Could you check a few things on this model? Use its own coordinates, in mm. Round coordinates to 2 decimals unless told otherwise and drop trailing zeros. Order: outer loops, then holes, each group sorted by start corner. A loop starts at its lowest first (then second) coordinate and runs counter-clockwise, first axis right, second up. Notation, with made-up numbers: M 24,11 L 31,11 A18 cw 31,22 Z; hole C -38,31.25 d11. An arc over 180 degrees is marked long. Write each question's results on one line, items separated by ' | '. Start each with the question number.
1. Suppose I cut it at D-D on x = 28. Write out the boundary of the cut face in (y, z).
2. We'd pull the mould along Z, two halves only. Please class faces 1 (the flat face through (15, -1.626, -13)), 2 (the flat face through (59.822, 0.023, 34.384)), 3 (the cylindrical face through (-11.59, 0.02, -15.12)): released by +Z, released by -Z, zero draft, split by the parting line, or undercut.
3. Please list where these lines run through material, in increasing order: L1, parallel to X at y = -0.35, z = 0; L2, parallel to X at y = -1.05, z = 10.5; L3, parallel to X at y = 0.15, z = -53.
4. I'm going to push a flat-ended pin straight in: pin 1 (1 mm diameter, centred on y = 1.5, z = -41, fed in from +X). Where does the tip first touch, or does it pass through?
5. Suppose I cut it at C-C on z = -17.5. Write out the boundary of the cut face in (x, y), and give its area (3 significant figures).
6. Suppose I cut it at A-A on x = 0. Write out the boundary of the cut face in (y, z).
7. Suppose I cut it at B-B on y = -0.45. Write out the boundary of the cut face in (x, z) (3 decimals).
from build123d import *

# Parameters (mm, degrees)
BOSS_EXTRUDE1_DEPTH = 1.6256
SKETCH3_R           = 19.05
CUT_EXTRUDE2_DEPTH  = 95.519790354


with BuildPart() as part:
    # Sketch1 → Boss-Extrude1 (new, symmetric)
    with BuildSketch(Plane(origin=(0, 0, 0), x_dir=(1, 0, 0), z_dir=(0, 1, 0))):
        with BuildLine():
            ThreePointArc((-64.51761314, -26.250738686), (-26.175423514, 15.112387812), (-9.525, 68.999261314))
            Line((-9.525, 68.999261314), (-9.525, 5.499261314))
            Line((-9.525, 5.499261314), (-64.51761314, -26.250738686))
        make_face()
        Polygon((-9.525, 5.499261314), (-9.525, 68.999261314), (9.525, 68.999261314), (9.525, 5.499261314), (64.51761314, -26.250738686), (54.99261314, -42.748522628), (0, -10.998522628), (-54.99261314, -42.748522628), (-64.51761314, -26.250738686), align=None)
        with BuildLine():
            ThreePointArc((54.99261314, -42.748522628), (0, -30.224775624), (-54.99261314, -42.748522628))
            Line((-54.99261314, -42.748522628), (0, -10.998522628))
            Line((0, -10.998522628), (54.99261314, -42.748522628))
        make_face()
        with BuildLine():
            ThreePointArc((9.525, 68.999261314), (26.175423514, 15.112387812), (64.51761314, -26.250738686))
            Line((64.51761314, -26.250738686), (9.525, 5.499261314))
            Line((9.525, 5.499261314), (9.525, 68.999261314))
        make_face()
    extrude(amount=BOSS_EXTRUDE1_DEPTH, both=True)

    # Sketch3 → Cut-Extrude2 (cut, through all)
    with BuildSketch(Plane(origin=(0, 1.6256, 0), x_dir=(1, 0, 0), z_dir=(0, 1, 0))):
        with Locations(Location((0, 0, 0), (0, 0, 270))):
            Circle(SKETCH3_R)
    extrude(amount=-CUT_EXTRUDE2_DEPTH, mode=Mode.SUBTRACT)


solid = part.part
Filled sheet:
1) outline: M -1.63,-12.05 L 1.63,-12.05 L 1.63,33.35 L -1.63,33.35 Z
2) face 1: zero draft | face 2: released by +Z | face 3: undercut
3) L1: x = -36.42 to -19.05, 19.05 to 36.42 | L2: x = -45.67 to -15.9, 15.9 to 45.67 | L3: x = -11.77 to 11.77
4) pin 1: stops at x = 15.01
5) outline: M -24.83,-1.63 L -7.53,-1.63 L -7.53,1.63 L -24.83,1.63 Z; M 7.53,-1.63 L 24.83,-1.63 L 24.83,1.63 L 7.53,1.63 Z | area: 113 mm^2
6) outline: M -1.63,-69 L 1.63,-69 L 1.63,-19.05 L -1.63,-19.05 Z; M -1.63,19.05 L 1.63,19.05 L 1.63,30.22 L -1.63,30.22 Z
7) outline: M -64.518,26.251 A127 cw -9.525,-68.999 L 9.525,-68.999 A127 cw 64.518,26.251 L 54.993,42.749 A127 cw -54.993,42.749 Z; hole C 0,0 d38.1
